Check sheet for the modelled part. Datum: model origin and axes. Units: mm. A direction names the side the tool comes from. Give positions to 0.01 mm unless a question says otherwise; leave off trailing zeros. Order: outer loops, then holes, each group sorted by start corner. A loop starts at its lowest first (then second) coordinate and runs counter-clockwise, first axis right, second up.
Item 1: Sectioned sample at B-B on y = 22. Record the boundary of the cut face in (x, z), and give its area (3 significant figures).
Item 2: Sectioned sample at A-A on x = 79. Record the boundary of the cut face in (y, z), and give its area (3 significant figures).
Item 3: Sectioned sample at D-D on z = 46. Record the boundary of the cut face in (x, y), and give its area (3 significant figures).
Item 4: Sectioned sample at C-C on z = 32. Record the boundary of the cut face in (x, y).
Item 5: Release check for a two-part mould opening along Y. For faces 5 (the flat face through (79, 17, 2)), 6 (the flat face through (79, 27, 2)), 7 (the cylindrical face through (-5.221, 23.686, 2.465)) record: released by +Y, released by -Y, zero draft, split by the parting line, or undercut.
Item 6: Material ranges on line 1 along Y through (x, z) = (42, 17); line 2 along Y through (x, z) = (4.5, 21); line 3 along X through (y, z) = (22, 3.65), recorded low to high.
Item 7: Gauge pin test, flat ends, axial feed: P1, Ø2.5, axis at x = -6, z = 1.5, coming from the +Y side; P2, Ø3, axis at y = 20, z = 18.5, coming from the -X side; P3, Ø5, axis at x = 30.5, y = 10.5, coming from the -Z side; P4, Ø0.6, axis at y = 30.5, z = 12, coming from the +X side. Record the tip position at first contact, or that the pin passes through.
Item 8: Access from +Z, -Z, +X, -X, +Y, -Y to the whole of each face (thin tool, end or side, straight path). Record for faces 1 (the flat face through (62, 31, 3)), 2 (the flat face through (-5, 27, 2)), 3 (the flat face through (81, 22, 5)), 4 (the flat face through (0, 37, 2)).
from build123d import *

# Parameters (mm, degrees)
BOX003_W          = 6
BOX003_H          = 6
BOX003_DEPTH      = 21
BOX004_W          = 12
BOX004_H          = 5
BOX004_DEPTH      = 27
CYLINDER003_R     = 1.7
CYLINDER003_DEPTH = 10
CYLINDER005_R     = 1.7
CYLINDER005_DEPTH = 10
CYLINDER007_R     = 1.7
CYLINDER007_DEPTH = 10
CYLINDER001_R     = 1.7
CYLINDER001_DEPTH = 10
BOX001_W          = 71
BOX001_H          = 45
BOX001_DEPTH      = 50
BOX_W             = 76
BOX_H             = 50
BOX_DEPTH         = 50
CYLINDER009_R     = 1.7
CYLINDER009_DEPTH = 10
BOX006_W          = 10
BOX006_H          = 10
BOX006_DEPTH      = 5
CYLINDER008_R     = 1.7
CYLINDER008_DEPTH = 10
BOX005_W          = 10
BOX005_H          = 10
BOX005_DEPTH      = 5
CYLINDER002_R     = 3
CYLINDER002_DEPTH = 50
CYLINDER004_R     = 3
CYLINDER004_DEPTH = 50
CYLINDER006_R     = 3
CYLINDER006_DEPTH = 50
CYLINDER_R        = 3
CYLINDER_DEPTH    = 50
BOX002_W          = 74
BOX002_H          = 2
BOX002_DEPTH      = 27
CHAMFER_SIZE      = 1
CHAMFER002_SIZE   = 1
FILLET_R          = 4
CHAMFER003_SIZE   = 1
FILLET007_1_R     = 2
FILLET007_2_R     = 1


with BuildPart() as obj1:
    # Box003 → Box003 (new body)
    with BuildSketch(Plane(origin=(-3, 34, 2), x_dir=(1, 0, 0), z_dir=(0, 0, 1))):
        with Locations((3, 3)):
            Rectangle(BOX003_W, BOX003_H)
    extrude(amount=BOX003_DEPTH)


with BuildPart() as obj2:
    # Box004 → Box004 (new body)
    with BuildSketch(Plane(origin=(56, 28, 3), x_dir=(1, 0, 0), z_dir=(0, 0, 1))):
        with Locations((6, 2.5)):
            Rectangle(BOX004_W, BOX004_H)
    extrude(amount=BOX004_DEPTH)


with BuildPart() as obj3:
    # Cylinder003 → Cylinder003 (new body)
    with BuildSketch(Plane(origin=(71, 3, 40), x_dir=(1, 0, 0), z_dir=(0, 0, 1))):
        Circle(CYLINDER003_R)
    extrude(amount=CYLINDER003_DEPTH)


with BuildPart() as obj4:
    # Cylinder005 → Cylinder005 (new body)
    with BuildSketch(Plane(origin=(3, 45, 40), x_dir=(1, 0, 0), z_dir=(0, 0, 1))):
        Circle(CYLINDER005_R)
    extrude(amount=CYLINDER005_DEPTH)


with BuildPart() as obj5:
    # Cylinder007 → Cylinder007 (new body)
    with BuildSketch(Plane(origin=(71, 45, 40), x_dir=(1, 0, 0), z_dir=(0, 0, 1))):
        Circle(CYLINDER007_R)
    extrude(amount=CYLINDER007_DEPTH)


with BuildPart() as obj6:
    # Cylinder001 → Cylinder001 (new body)
    with BuildSketch(Plane(origin=(3, 3, 40), x_dir=(1, 0, 0), z_dir=(0, 0, 1))):
        Circle(CYLINDER001_R)
    extrude(amount=CYLINDER001_DEPTH)

    # Fusion003: union obj3, obj4, obj5
    add(obj3.part)
    add(obj4.part)
    add(obj5.part)


with BuildPart() as vaciado_interior:
    # Box001 → Box001 (new body)
    with BuildSketch(Plane(origin=(1.5, 1.5, 1.5), x_dir=(1, 0, 0), z_dir=(0, 0, 1))):
        with Locations((35.5, 22.5)):
            Rectangle(BOX001_W, BOX001_H)
    extrude(amount=BOX001_DEPTH)


with BuildPart() as parte_inferior:
    # Box → Box (new body)
    with BuildSketch(Plane(origin=(-1, -1, 0), x_dir=(1, 0, 0), z_dir=(0, 0, 1))):
        with Locations((38, 25)):
            Rectangle(BOX_W, BOX_H)
    extrude(amount=BOX_DEPTH)

    # Cut: cut vaciado interior
    add(vaciado_interior.part, mode=Mode.SUBTRACT)


with BuildPart() as obj7:
    # Cylinder009 → Cylinder009 (new body)
    with BuildSketch(Plane(origin=(-5, 22, -1), x_dir=(1, 0, 0), z_dir=(0, 0, 1))):
        Circle(CYLINDER009_R)
    extrude(amount=CYLINDER009_DEPTH)


with BuildPart() as cut002:
    # Box006 → Box006 (new body)
    with BuildSketch(Plane(origin=(-10, 17, 0), x_dir=(1, 0, 0), z_dir=(0, 0, 1))):
        with Locations((5, 5)):
            Rectangle(BOX006_W, BOX006_H)
    extrude(amount=BOX006_DEPTH)

    # Cut002: cut obj7
    add(obj7.part, mode=Mode.SUBTRACT)


with BuildPart() as cut002_1:
    # Cut002 placement: moved
    add(cut002.part.moved(Location((84, 0, 0))))


with BuildPart() as obj8:
    # Cylinder008 → Cylinder008 (new body)
    with BuildSketch(Plane(origin=(-5, 22, -1), x_dir=(1, 0, 0), z_dir=(0, 0, 1))):
        Circle(CYLINDER008_R)
    extrude(amount=CYLINDER008_DEPTH)


with BuildPart() as obj9:
    # Box005 → Box005 (new body)
    with BuildSketch(Plane(origin=(-10, 17, 0), x_dir=(1, 0, 0), z_dir=(0, 0, 1))):
        with Locations((5, 5)):
            Rectangle(BOX005_W, BOX005_H)
    extrude(amount=BOX005_DEPTH)

    # Cut001: cut obj8
    add(obj8.part, mode=Mode.SUBTRACT)

    # Fusion: union Cut002
    add(cut002_1.part)


with BuildPart() as soporte_tornillo001:
    # Cylinder002 → Cylinder002 (new body)
    with BuildSketch(Plane(origin=(71, 3, 0), x_dir=(1, 0, 0), z_dir=(0, 0, 1))):
        Circle(CYLINDER002_R)
    extrude(amount=CYLINDER002_DEPTH)


with BuildPart() as soporte_tornillo002:
    # Cylinder004 → Cylinder004 (new body)
    with BuildSketch(Plane(origin=(3, 45, 0), x_dir=(1, 0, 0), z_dir=(0, 0, 1))):
        Circle(CYLINDER004_R)
    extrude(amount=CYLINDER004_DEPTH)


with BuildPart() as soporte_tornillo003:
    # Cylinder006 → Cylinder006 (new body)
    with BuildSketch(Plane(origin=(71, 45, 0), x_dir=(1, 0, 0), z_dir=(0, 0, 1))):
        Circle(CYLINDER006_R)
    extrude(amount=CYLINDER006_DEPTH)


with BuildPart() as obj10:
    # Cylinder → Cylinder (new body)
    with BuildSketch(Plane(origin=(3, 3, 0), x_dir=(1, 0, 0), z_dir=(0, 0, 1))):
        Circle(CYLINDER_R)
    extrude(amount=CYLINDER_DEPTH)

    # Fusion001: union soporte tornillo001, soporte tornillo002, soporte tornillo003
    add(soporte_tornillo001.part)
    add(soporte_tornillo002.part)
    add(soporte_tornillo003.part)


with BuildPart() as parte_inferior001:
    # Box002 → Box002 (new body)
    with BuildSketch(Plane(origin=(0, 30, 0), x_dir=(1, 0, 0), z_dir=(0, 0, 1))):
        with Locations((37, 1)):
            Rectangle(BOX002_W, BOX002_H)
    extrude(amount=BOX002_DEPTH)

    # Fusion002: union parte inferior, obj9, obj10
    add(parte_inferior.part)
    add(obj9.part)
    add(obj10.part)

    # Cut003: cut obj6
    add(obj6.part, mode=Mode.SUBTRACT)

    # Cut004: cut obj2
    add(obj2.part, mode=Mode.SUBTRACT)

    # Cut005: cut obj1
    add(obj1.part, mode=Mode.SUBTRACT)

    # Chamfer
    chamfer_edges = [parte_inferior001.edges().sort_by_distance(p)[0] for p in [
        (72.5, 17.799038, 1.5),
    ]]
    chamfer(chamfer_edges, length=CHAMFER_SIZE)

    # Chamfer002
    chamfer002_edges = [parte_inferior001.edges().sort_by_distance(p)[0] for p in [
        (-1, 27, 2.5),
    ]]
    chamfer(chamfer002_edges, length=CHAMFER002_SIZE)

    # Fillet
    fillet_edges = [parte_inferior001.edges().sort_by_distance(p)[0] for p in [
        (-1, 49, 25),
        (-1, -1, 25),
        (75, 49, 25),
        (75, -1, 25),
    ]]
    fillet(fillet_edges, radius=FILLET_R)

    # Chamfer003
    chamfer003_edges = [parte_inferior001.edges().sort_by_distance(p)[0] for p in [
        (-1, 22, 5),
        (-1, 17, 2.5),
        (75, 17, 2.5),
        (75, 27, 2.5),
        (75, 22, 5),
        (72.5, 30, 14.75),
        (72.5, 31, 27),
        (72.5, 32, 14.25),
        (1.5, 30, 14.25),
        (1.5, 31, 27),
        (1.5, 32, 14.25),
    ]]
    chamfer(chamfer003_edges, length=CHAMFER003_SIZE)

    # Fillet007 1
    fillet007_1_edges = [parte_inferior001.edges().sort_by_distance(p)[0] for p in [
        (0.25, 40, 23),
        (0.25, 34, 23),
        (84, 27, 2.5),
        (84, 17, 2.5),
        (-10, 27, 2.5),
        (-10, 17, 2.5),
    ]]
    fillet(fillet007_1_edges, radius=FILLET007_1_R)

    # Fillet007 2
    fillet007_2_edges = [parte_inferior001.edges().sort_by_distance(p)[0] for p in [
        (68, 31, 27),
        (56, 31, 27),
    ]]
    fillet(fillet007_2_edges, radius=FILLET007_2_R)


solid = parte_inferior001.part
Report:
1. outline: (-10, 0) - (-6.7, 0) - (-6.7, 5) - (-10, 5) - close; (-3.3, 0) - (77.3, 0) - (77.3, 5) - (76, 5) - (75, 6) - (75, 50) - (72.5, 50) - (72.5, 2.5) - (71.5, 1.5) - (1.5, 1.5) - (1.5, 50) - (-1, 50) - (-1, 6) - (-2, 5) - (-3.3, 5) - close; (80.7, 0) - (84, 0) - (84, 5) - (80.7, 5) - close
1. area: 414 mm2
2. outline: (17, 0) - (20.3, 0) - (20.3, 5) - (17, 5) - close; (23.7, 0) - (27, 0) - (27, 5) - (23.7, 5) - close
2. area: 33.0 mm2
3. outline: (-1, 3) arc R4 ccw to (3, -1) - (71, -1) arc R4 ccw to (75, 3) - (75, 45) arc R4 ccw to (71, 49) - (3, 49) arc R4 ccw to (-1, 45) - close; hole circle Ø3.4 at (3, 3); hole circle Ø3.4 at (3, 45); hole (1.5, 5.6) arc R3 cw to (5.6, 1.5) - (68.4, 1.5) arc R3 cw to (72.5, 5.6) - (72.5, 42.4) arc R3 cw to (68.4, 46.5) - (5.6, 46.5) arc R3 cw to (1.5, 42.4) - close; hole circle Ø3.4 at (71, 3); hole circle Ø3.4 at (71, 45)
3. area: 627 mm2
4. outline: (-1, 3) arc R4 ccw to (3, -1) - (71, -1) arc R4 ccw to (75, 3) - (75, 45) arc R4 ccw to (71, 49) - (3, 49) arc R4 ccw to (-1, 45) - close; hole (1.5, 5.6) arc R3 cw to (5.6, 1.5) - (68.4, 1.5) arc R3 cw to (72.5, 5.6) - (72.5, 42.4) arc R3 cw to (68.4, 46.5) - (5.6, 46.5) arc R3 cw to (1.5, 42.4) - close
5. face 5: released by -Y
5. face 6: released by +Y
5. face 7: undercut
6. line 1: y = -1 to 1.5, 30 to 32, 46.5 to 49
6. line 2: y = -1 to 5.6, 30 to 32, 42.4 to 49
6. line 3: x = -10 to -6.7, -3.3 to 1.5, 72.5 to 77.3, 80.7 to 84
7. P1: stops at y = 27
7. P2: stops at x = -1
7. P3: stops at z = 0
7. P4: stops at x = 75
8. face 1: +Z
8. face 2: +Z, -Z, -X, +Y
8. face 3: +Z, +X, +Y, -Y
8. face 4: -X
